For this review, take the finished solid that the model builds, in its own axes (mm). A direction names the side the tool comes from. Coordinates: 2 decimals unless noted, no trailing zeros. Loops run counter-clockwise (first coordinate to the right, second up) from the corner with the lowest first, then second, coordinate; pieces in that order, holes last. Notation, with made-up numbers: M -37,39 L 22,39 A24 cw 22,62 Z; hole C -12.75,-12 d4. An arc over 180 degrees is marked long. Use one line per item in the form item = value.
```python
from build123d import *

# Parameters (mm, degrees)
BOSS_EXTRUDE1_DEPTH = 25.4
CUT_EXTRUDE1_DEPTH  = 5.08
SKETCH3_OUTSIDE_W   = 13.788
SKETCH3_OUTSIDE_H   = 14.77
SKETCH3_OUTSIDE_R   = 3.175
CUT_EXTRUDE2_DEPTH  = 13.7


with BuildPart() as part:
    # Sketch1 → Boss-Extrude1 (new body)
    with BuildSketch(Plane.XY):
        Polygon((0, 3.666174209), (-3.175, 1.833087105), (-3.175, -1.833087105), (0, -3.666174209), (3.175, -1.833087105), (3.175, 1.833087105), align=None)
    extrude(amount=-BOSS_EXTRUDE1_DEPTH)

    # Sketch2 → Cut-Extrude1 (cut)
    with BuildSketch(Plane.XY):
        with BuildLine():
            Line((-0.756832981, -1.278711324), (1.485812981, 0.016080926))
            ThreePointArc((1.485812981, 0.016080926), (-0.74295, 1.286827147), (-0.756832981, -1.278711324))
        make_face()
    extrude(amount=-CUT_EXTRUDE1_DEPTH, mode=Mode.SUBTRACT)

    # Sketch3 outside → Cut-Extrude2 (cut, through all)
    with BuildSketch(Plane.XY.offset(-12.7)):
        Rectangle(SKETCH3_OUTSIDE_W, SKETCH3_OUTSIDE_H)
        Circle(SKETCH3_OUTSIDE_R, mode=Mode.SUBTRACT)
    extrude(amount=-CUT_EXTRUDE2_DEPTH, mode=Mode.SUBTRACT)


solid = part.part
```
1. Consider section A-A on z = -2.75. Write out the cut boundary in (x, y) (3 decimals).
Computed values:
outline = M -3.175,-1.833 L 0,-3.666 L 3.175,-1.833 L 3.175,1.833 L 0,3.666 L -3.175,1.833 Z; hole M -0.757,-1.279 L 1.486,0.016 A1.486 ccw long Z
2. Wall thickness on line 1 along Z through (x, y) = (-3, -1.25); line 2 along Z through (x, y) = (-0.75, -1); line 3 along X through (y, z) = (0, -1.5) (3 decimals): over which ranges is each line inside the solid? List them lowest first. Write a range as from..to.
Computed values:
line_1 = -12.7..0
line_2 = -25.4..-5.08
line_3 = -3.175..-1.486, 1.458..3.175
3. Consider section B-B on y = 0.5. Write out the cut boundary in (x, z) (3 decimals).
Computed values:
outline = M -3.175,-12.7 L -3.135,-12.7 L -3.135,-25.4 L 3.135,-25.4 L 3.135,-12.7 L 3.175,-12.7 L 3.175,0 L 1.399,0 L 1.399,-5.08 L -1.399,-5.08 L -1.399,0 L -3.175,0 Z
4. Consider section D-D on z = -8. Write out the cut boundary in (x, y) (3 decimals).
Computed values:
outline = M -3.175,-1.833 L 0,-3.666 L 3.175,-1.833 L 3.175,1.833 L 0,3.666 L -3.175,1.833 Z
5. Tool access review of faces 1 (the face through (0, 0, -5.08)), 2 (the face through (-0.01, -3.34, -12.7)), 3 (the face through (-0.69, -3.1, -18.96)), 4 (the face through (2.9, -1.7, -12.7)), 5 (the face through (2.9, 1.7, -12.7)): name each direction out of +Z, -Z, +X, -X, +Y, -Y from which nothing blocks a thin tool from reaching the whole face with its end or side.
Computed values:
face_1 = +Z
face_2 = -Z, -Y
face_3 = -Z
face_4 = -Z, +X, -Y
face_5 = -Z, +X, +Y
6. For pin 1 Ø1.5 at (y, z) = (3, -11) entering from +X; pin 2 Ø2 at (y, z) = (1.5, -15.5) entering from -X, all flat-tipped, find the tip position at first contact; note any pin that passes through.
Computed values:
pin_1 = 2.45
pin_2 = -3.14
7. Draft analysis for pull direction Y (two halves, no side actions). For faces 6 (the face through (0, 3.4, -12.7)), 7 (the face through (-1.57, 2.76, -6.26)), 8 (the face through (0.35, -0.64, -2.5)), state which applies: +Y half, -Y half, draft (parallel to the pull), parting line (faces both ways), or undercut.
Computed values:
face_6 = draft
face_7 = +Y half
face_8 = undercut
8. Consider section C-C on x = -2. Write out the cut boundary in (y, z), plus the area to 3 significant figures.
Computed values:
outline = M -2.51,-12.7 L -2.47,-12.7 L -2.47,-25.4 L 2.47,-25.4 L 2.47,-12.7 L 2.51,-12.7 L 2.51,0 L -2.51,0 Z
area = 126 mm2
